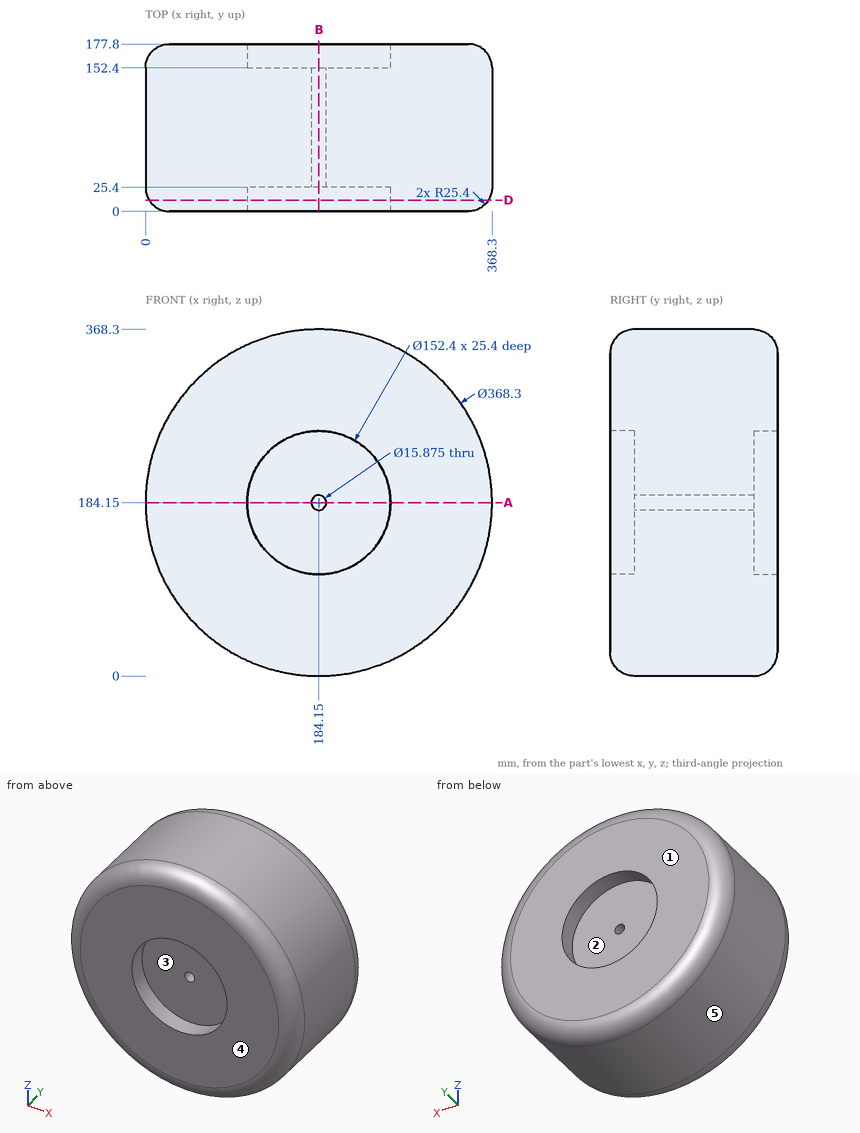
Job drawing, mm, ordinate dimensions from the low corner. One solid piece. A direction names the side the tool comes from. Give positions to 0.01 mm unless a question says otherwise; leave off trailing zeros. Order: outer loops, then holes, each group sorted by start corner. A loop starts at its lowest first (then second) coordinate and runs counter-clockwise, first axis right, second up. Notation, with made-up numbers: (70.25, 80.5) - (105.25, 80.5) arc R13 ccw to (105.25, 105.5) - close; hole circle Ø2 at (89.5, 21.5). An arc over 180 degrees is marked (long way). One line per question, with ' | ' between items.
1. Band-saw the part on D-D on y = 12. List the corners of the cut face in (x, z).
Filled in:
outline: circle Ø360.66 at (184.15, 184.15); hole circle Ø152.4 at (184.15, 184.15)
2. Drop flat-ended pins along their axis: P1, Ø12.5, axis at x = 184.15, z = 184.15, coming from the -Y side; P2, Ø10, axis at y = 69, z = 46, coming from the -X side; P3, Ø4, axis at y = 72, z = 93, coming from the -X side; P4, Ø4, axis at x = 229, y = 119, coming from the -Z side. Give the stop position or say it passes through.
Filled in:
P1: through | P2: x = 56.94 | P3: x = 23.02 | P4: z = 5.05
3. Band-saw the part on A-A on z = 184.15. List the corners of the cut face in (x, y), then the cut area to 3 significant figures.
Filled in:
outline: (0, 25.4) arc R25.4 ccw to (25.4, 0) - (107.95, 0) - (107.95, 25.4) - (176.21, 25.4) - (176.21, 152.4) - (107.95, 152.4) - (107.95, 177.8) - (25.4, 177.8) arc R25.4 ccw to (0, 152.4) - close; (192.09, 25.4) - (260.35, 25.4) - (260.35, 0) - (342.9, 0) arc R25.4 ccw to (368.3, 25.4) - (368.3, 152.4) arc R25.4 ccw to (342.9, 177.8) - (260.35, 177.8) - (260.35, 152.4) - (192.09, 152.4) - close | area: 55,200 mm²
4. Which spindle directions (+Z, -Z, +X, -X, +Y, -Y) get a long thin tool onto all of the face, cutting with end or side? Do the marked faces 1 and 2. Say none if no direction does.
Filled in:
face 1: +Z, -Z, +X, -X, +Y | face 2: +Y
5. Pull direction X, two halves, no side cores. Call the marked faces 3, 4 and 5: +X half, -X half, draft (parallel to the pull), parting line (faces both ways), or undercut.
Filled in:
face 3: undercut | face 4: draft | face 5: parting line
6. Band-saw the part on B-B on x = 184.15. List the corners of the cut face in (y, z), then the cut area to 3 significant figures.
Filled in:
outline: (0, 25.4) arc R25.4 ccw to (25.4, 0) - (152.4, 0) arc R25.4 ccw to (177.8, 25.4) - (177.8, 107.95) - (152.4, 107.95) - (152.4, 176.21) - (25.4, 176.21) - (25.4, 107.95) - (0, 107.95) - close; (0, 260.35) - (25.4, 260.35) - (25.4, 192.09) - (152.4, 192.09) - (152.4, 260.35) - (177.8, 260.35) - (177.8, 342.9) arc R25.4 ccw to (152.4, 368.3) - (25.4, 368.3) arc R25.4 ccw to (0, 342.9) - close | area: 55,200 mm²
7. Drill centre lines: probe 1 along Z at (x, y) = (184, 99); probe 2 along Z at (x, y) = (135.5, 7); probe 3 along X at (y, z) = (10, 184). Where is each one in solid material? Low to high.
Filled in:
probe 1: 0 to 176.21, 192.09 to 368.3 | probe 2: 14.74 to 125.5, 242.8 to 353.56 | probe 3: 5.2 to 107.95, 260.35 to 363.1
